from build123d import *

# Parameters (mm, degrees)
SKETCH011_W             = 50
SKETCH011_H             = 50
PAD001_DEPTH            = 25
FILLET001_R             = 3
POCKET004_DEPTH         = 20
SKETCH013_W             = 42
SKETCH013_H             = 40
POCKET003_DEPTH         = 4
SKETCH010_W             = 40
SKETCH010_H             = 40
POCKET005_DEPTH         = 1
BODY001_PLACEMENT_ANGLE = 180


with BuildPart() as part:
    # Sketch011 → Pad001 (new body)
    with BuildSketch(Plane.XY):
        Rectangle(SKETCH011_W, SKETCH011_H)
    extrude(amount=PAD001_DEPTH)

    # Fillet001
    fillet001_edges = [part.edges().sort_by_distance(p)[0] for p in [
        (0, -25, 0),
        (-25, 0, 0),
        (0, 25, 0),
        (25, 0, 0),
        (-25, -25, 12.5),
        (25, 25, 12.5),
        (-25, 25, 12.5),
        (25, -25, 12.5),
    ]]
    fillet(fillet001_edges, radius=FILLET001_R)

    # Sketch012 (on Face2 of Fillet001) → Pocket004 (cut)
    with BuildSketch(Plane.XY.offset(25)):
        Polygon((-20, 25), (-20, 24), (-22, 24), (-22, 22.3), (-20, 22.3), (-20, 20), (-22.3, 20), (-22.3, 22), (-24, 22), (-24, 20), (-25, 20), (-25, -20), (-24, -20), (-24, -22), (-22.3, -22), (-22.3, -20), (-20, -20), (-20, -22.3), (-22, -22.3), (-22, -24), (-20, -24), (-20, -25), (20, -25), (20, -24), (22, -24), (22, -22.3), (20, -22.3), (20, -20), (22.3, -20), (22.3, -22), (24, -22), (24, -20), (25, -20), (25, 20), (24, 20), (24, 22), (22.3, 22), (22.3, 20), (20, 20), (20, 22.3), (22, 22.3), (22, 24), (20, 24), (20, 25), align=None)
    extrude(amount=-POCKET004_DEPTH, mode=Mode.SUBTRACT)

    # Sketch013 (on Face7 of Pocket004) → Pocket003 (cut)
    with BuildSketch(Plane.XY.offset(5)):
        Rectangle(SKETCH013_W, SKETCH013_H)
    extrude(amount=-POCKET003_DEPTH, mode=Mode.SUBTRACT)

    # Sketch010 (on Face47 of Pocket003) → Pocket005 (cut)
    with BuildSketch(Plane.XY.offset(1)):
        Rectangle(SKETCH010_W, SKETCH010_H)
    extrude(amount=-POCKET005_DEPTH, mode=Mode.SUBTRACT)


with BuildPart() as part_1:
    # Body001 placement: moved
    add(part.part.moved(Location((0, 0, 50))).rotate(Axis((0, 0, 50), (0, 1, 0)), BODY001_PLACEMENT_ANGLE))


solid = part_1.part
Work out the finished part from the listing and answer in its coordinate system (mm). A direction names the side the tool comes from. Coordinates: 2 decimals unless noted, no trailing zeros. Loops run counter-clockwise (first coordinate to the right, second up) from the corner with the lowest first, then second, coordinate; pieces in that order, holes last. Notation, with made-up numbers: (-11.5, -16) -> (-5.5, -16) arc R23 cw to (-5.5, 15) -> close; hole circle Ø4 at (-31, 46.5). An arc over 180 degrees is marked (long way). Answer as CSV lines item,"result".
1) Flat-ended cylindrical pins translate along their axes: pin 1 (0.8 mm diameter, centred on x = -20.5, y = 3.5, fed in from -Z); pin 2 (0.5 mm diameter, centred on x = 24.5, z = 31.5, fed in from +Y); pin 3 (0.5 mm diameter, centred on x = -23, z = 33.5, fed in from +Y). Find the tip coordinate at first contact, or state that the pin passes through.
A:
pin 1,"stops at z = 49"
pin 2,"stops at y = 23.98"
pin 3,"stops at y = 24.9"
2) Straight lines are drawn through the part: probe 1 along Y at (x, z) = (-11.5, 46); probe 2 along X at (y, z) = (-11, 47.25); probe 3 along Z at (x, y) = (-8, -22). For each, find the intervals that lie inside material, in ascending order.
A:
probe 1,"y = -25 to -20, 20 to 25"
probe 2,"x = -24.99 to -21, 21 to 24.99"
probe 3,"z = 45 to 50"
3) The part is cut by section A-A (y = 15). Give the vertices of the cut face in (x, z).
A:
outline,"(-25, 45) -> (-21, 45) -> (-21, 49) -> (-20, 49) -> (-20, 50) -> (-22, 50) arc R3 ccw to (-25, 47) -> close; (20, 49) -> (21, 49) -> (21, 45) -> (25, 45) -> (25, 47) arc R3 ccw to (22, 50) -> (20, 50) -> close"
4) The part is cut by section D-D (z = 31.5). State how many separate pieces and enclosed holes the cut face has, and give its area (3 significant figures).
A:
separate pieces,"4"
enclosed holes,"0"
area,"65.1 mm²"
5) For faces 1 (the face through (-24.14, 0.31, 49.1)), 2 (the face through (-21, -24, 35)), 3 (the face through (-20, 21, 35)), determine the directions among +Z, -Z, +X, -X, +Y, -Y from which every point of the face is accessible in a straight line to the end or side of a thin tool.
A:
face 1,"+Z, -X, +Y, -Y"
face 2,"-Z"
face 3,"-Z, +Y, -Y"
6) The part is cut by section C-C (z = 48). Give the vertices of the cut face in (x, y).
A:
outline,"(-24.83, -22) arc R2.83 ccw to (-22, -24.83) -> (22, -24.83) arc R2.83 ccw to (24.83, -22) -> (24.83, 22) arc R2.83 ccw to (22, 24.83) -> (-22, 24.83) arc R2.83 ccw to (-24.83, 22) -> close; hole (-21, -20) -> (21, -20) -> (21, 20) -> (-21, 20) -> close"
7) For a pull along Y with two mould halves and no side action, classify faces 4 (the face through (-24, -21, 35)), 5 (the face through (-24.14, 24.1, 35.85)), 6 (the face through (24.14, -24.1, 35.85)) as released by +Y, released by -Y, zero draft, split by the parting line, or undercut.
A:
face 4,"undercut"
face 5,"released by +Y"
face 6,"released by -Y"
8) The part is cut by section B-B (x = -13.5). Give the vertices of the cut face in (y, z), and give its area (3 significant figures).
A:
outline,"(-25, 45) -> (-20, 45) -> (-20, 50) -> (-22, 50) arc R3 ccw to (-25, 47) -> close; (20, 45) -> (25, 45) -> (25, 47) arc R3 ccw to (22, 50) -> (20, 50) -> close"
area,"46.1 mm²"
